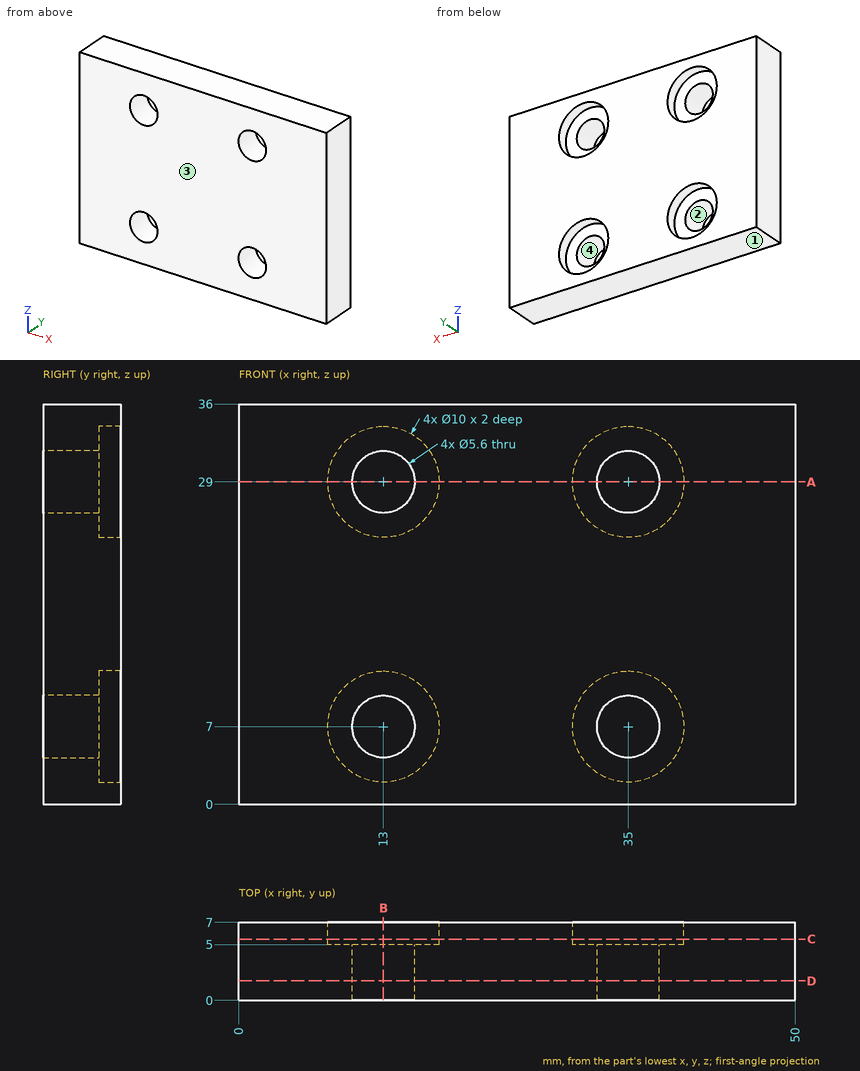
Print and shaded views of the part. All mm, measured from the part's lowest x, y and z. Coordinates: 2 decimals unless noted, no trailing zeros. Loops run counter-clockwise (first coordinate to the right, second up) from the corner with the lowest first, then second, coordinate; pieces in that order, holes last. Notation, with made-up numbers: (54.5, 66.25) - (84.5, 66.25) arc R32 cw to (84.5, 93.25) - close; hole circle Ø5 at (-8.75, 1.5). An arc over 180 degrees is marked (long way). Write item = value, one per line. Start each with the question number.
Item 1: Wall check: probe 1 along X at (y, z) = (2.05, 7); probe 2 along X at (y, z) = (5.6, 29); probe 3 along Z at (x, y) = (12.5, 2.5) (3 decimals). Give the ranges that are in metal, low to high. Write a range as [from, to].
Item 2: Pull direction Z, two halves, no side cores. Call the marked faces 1, 2, 3 and 4: +Z half, -Z half, draft (parallel to the pull), parting line (faces both ways), or undercut.
Item 3: Drop flat-ended pins along their axis: pin 1 Ø7.5 at (x, z) = (13, 29) entering from +Y; pin 2 Ø6.5 at (x, z) = (35, 7) entering from -Y; pin 3 Ø3.5 at (x, z) = (13, 7) entering from -Y. Give the stop position or say it passes through.
Item 4: Saw through at C-C, the plane y = 5.5. List the corners of the cut face in (x, z), then the cut area to 3 significant figures.
Item 5: Saw through at D-D, the plane y = 1.75. List the corners of the cut face in (x, z), then the cut area to 3 significant figures.
Item 6: Saw through at A-A, the plane z = 29. List the corners of the cut face in (x, y).
Item 7: Saw through at B-B, the plane x = 13. List the corners of the cut face in (y, z).
Answers:
q1.probe_1 = [0, 10.2], [15.8, 32.2], [37.8, 50]
q1.probe_2 = [0, 8], [18, 30], [40, 50]
q1.probe_3 = [0, 4.245], [9.755, 26.245], [31.755, 36]
q2.face_1 = -Z half
q2.face_2 = undercut
q2.face_3 = draft
q2.face_4 = undercut
q3.pin_1 = 5
q3.pin_2 = 0
q3.pin_3 = through
q4.outline = (0, 0) - (50, 0) - (50, 36) - (0, 36) - close; hole circle Ø10 at (13, 7); hole circle Ø10 at (13, 29); hole circle Ø10 at (35, 7); hole circle Ø10 at (35, 29)
q4.area = 1,490 mm2
q5.outline = (0, 0) - (50, 0) - (50, 36) - (0, 36) - close; hole circle Ø5.6 at (13, 7); hole circle Ø5.6 at (13, 29); hole circle Ø5.6 at (35, 7); hole circle Ø5.6 at (35, 29)
q5.area = 1,700 mm2
q6.outline = (0, 0) - (10.2, 0) - (10.2, 5) - (8, 5) - (8, 7) - (0, 7) - close; (15.8, 0) - (32.2, 0) - (32.2, 5) - (30, 5) - (30, 7) - (18, 7) - (18, 5) - (15.8, 5) - close; (37.8, 0) - (50, 0) - (50, 7) - (40, 7) - (40, 5) - (37.8, 5) - close
q7.outline = (0, 0) - (7, 0) - (7, 2) - (5, 2) - (5, 4.2) - (0, 4.2) - close; (0, 9.8) - (5, 9.8) - (5, 12) - (7, 12) - (7, 24) - (5, 24) - (5, 26.2) - (0, 26.2) - close; (0, 31.8) - (5, 31.8) - (5, 34) - (7, 34) - (7, 36) - (0, 36) - close
